Check sheet for the drawn part. Datum: minimum x, y, z corner. Units: mm. Give positions to 0.01 mm unless a question says otherwise; leave off trailing zeros. Order: outer loops, then holes, each group sorted by start corner. A loop starts at its lowest first (then second) coordinate and runs counter-clockwise, first axis right, second up.
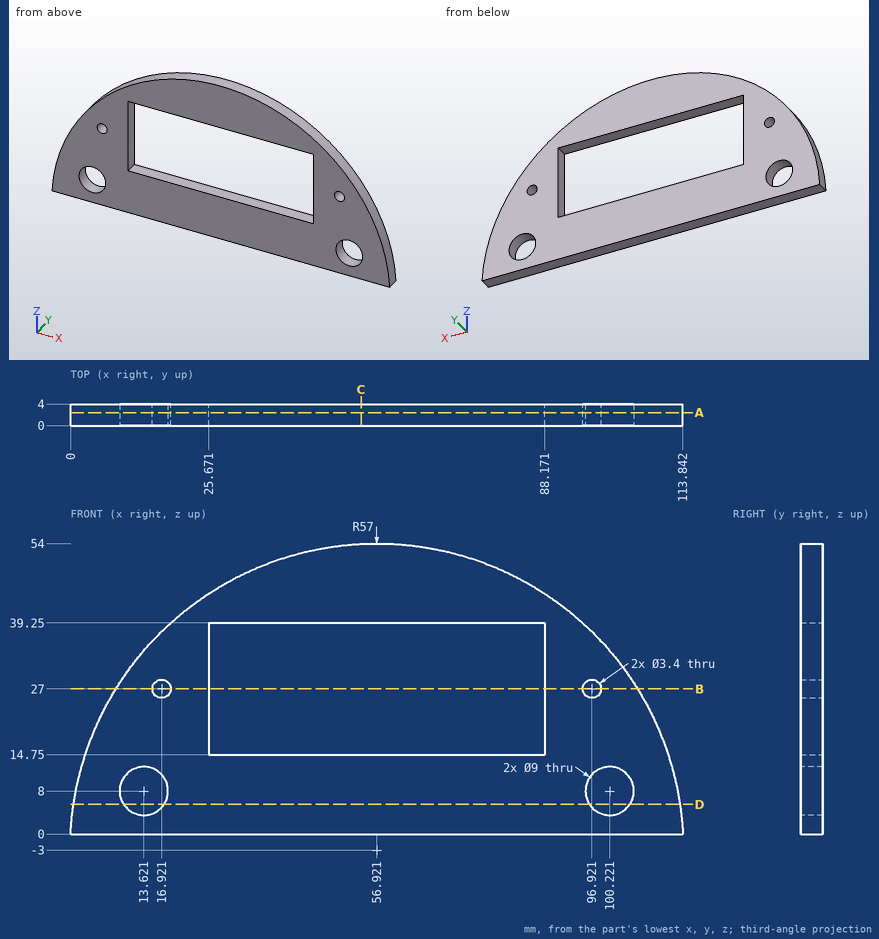
Q1. Sectioned sample at B-B, the plane z = 27. Record the cut outline in (x, y).
Q2. Material ranges on line 1 (Z direction, x = 35.5, y = 2.5); line 2 (X direction, y = 1.9, z = 25); line 3 (X direction, y = 2.1, z = 11), recorded low to high.
Q3. Sectioned sample at D-D, the plane z = 5.5. Record the cut outline in (x, y).
Q4. Sectioned sample at A-A, the plane y = 2.4. Record the cut outline in (x, z), plus the area to 3 significant figures.
Q5. Go/stop test with flat-tipped pins: P1, Ø1, axis at y = 3, z = 13, coming from the -X side; P2, Ø1.5, axis at x = 81.5, z = 16.5, coming from the -Y side; P3, Ø1, axis at y = 1, z = 16, coming from the +X side; P4, Ø2, axis at y = 1.5, z = 28, coming from the +X side. Record where each tip stops, or that it passes through.
Q6. Sectioned sample at C-C, the plane x = 54. Record the cut outline in (y, z).
Filled in:
1. outline: (8.45, 0) - (15.22, 0) - (15.22, 4) - (8.45, 4) - close; (18.62, 0) - (25.67, 0) - (25.67, 4) - (18.62, 4) - close; (88.17, 0) - (95.22, 0) - (95.22, 4) - (88.17, 4) - close; (98.62, 0) - (105.39, 0) - (105.39, 4) - (98.62, 4) - close
2. line 1: z = 0 to 14.75, 39.25 to 49.82
2. line 2: x = 7.27 to 25.67, 88.17 to 106.57
2. line 3: x = 1.67 to 10.27, 16.98 to 96.87, 103.58 to 112.17
3. outline: (0.56, 0) - (9.88, 0) - (9.88, 4) - (0.56, 4) - close; (17.36, 0) - (96.48, 0) - (96.48, 4) - (17.36, 4) - close; (103.96, 0) - (113.28, 0) - (113.28, 4) - (103.96, 4) - close
4. outline: (0, 0) - (113.84, 0) arc R57 ccw to start; hole circle Ø9 at (13.62, 8); hole circle Ø3.4 at (16.92, 27); hole (25.67, 14.75) - (88.17, 14.75) - (88.17, 39.25) - (25.67, 39.25) - close; hole circle Ø3.4 at (96.92, 27); hole circle Ø9 at (100.22, 8)
4. area: 3,090 mm2
5. P1: stops at x = 2.07
5. P2: passes through
5. P3: stops at x = 110.84
5. P4: stops at x = 105.39
6. outline: (0, 0) - (4, 0) - (4, 14.75) - (0, 14.75) - close; (0, 39.25) - (4, 39.25) - (4, 53.93) - (0, 53.93) - close
